```python
from build123d import *

# Parameters (mm, degrees)
SKETCH1_R           = 5
SKETCH1_R_2         = 1
BOSS_EXTRUDE1_DEPTH = 1
SKETCH3_R           = 6
BOSS_EXTRUDE2_DEPTH = 2
SKETCH4_R           = 5
CUT_EXTRUDE1_DEPTH  = 1
SKETCH5_R           = 4
CUT_EXTRUDE2_DEPTH  = 1
SKETCH6_R           = 3
BOSS_EXTRUDE3_DEPTH = 2
SKETCH7_R           = 1
CUT_EXTRUDE3_DEPTH  = 2


with BuildPart() as part:
    # Sketch1 → Boss-Extrude1 (new body)
    with BuildSketch(Plane(origin=(0, 0, 0), x_dir=(1, 0, 0), z_dir=(0, 1, 0))):
        with BuildLine():
            ThreePointArc((-4.117647059, 8.98545751), (-9.474873734, 9.474873734), (-8.98545751, 4.117647059))
            ThreePointArc((-8.98545751, 4.117647059), (-6.82182538, 0), (-8.98545751, -4.117647059))
            ThreePointArc((-8.98545751, -4.117647059), (-9.474873734, -9.474873734), (-4.117647059, -8.98545751))
            ThreePointArc((-4.117647059, -8.98545751), (0, -6.82182538), (4.117647059, -8.98545751))
            ThreePointArc((4.117647059, -8.98545751), (9.474873734, -9.474873734), (8.98545751, -4.117647059))
            ThreePointArc((8.98545751, -4.117647059), (6.82182538, 0), (8.98545751, 4.117647059))
            ThreePointArc((8.98545751, 4.117647059), (9.474873734, 9.474873734), (4.117647059, 8.98545751))
            ThreePointArc((4.117647059, 8.98545751), (0, 6.82182538), (-4.117647059, 8.98545751))
        make_face()
        with Locations(Location((0, 0, 0), (0, 0, 270))):
            Circle(SKETCH1_R, mode=Mode.SUBTRACT)
        with Locations(Location((-7, 7, 0), (0, 0, 270))):
            Circle(SKETCH1_R_2, mode=Mode.SUBTRACT)
        with Locations(Location((7, 7, 0), (0, 0, 270))):
            Circle(SKETCH1_R_2, mode=Mode.SUBTRACT)
        with Locations(Location((7, -7, 0), (0, 0, 270))):
            Circle(SKETCH1_R_2, mode=Mode.SUBTRACT)
        with Locations(Location((-7, -7, 0), (0, 0, 270))):
            Circle(SKETCH1_R_2, mode=Mode.SUBTRACT)
    extrude(amount=BOSS_EXTRUDE1_DEPTH)

    # Sketch3 → Boss-Extrude2 (add)
    with BuildSketch(Plane(origin=(0, 1, 0), x_dir=(1, 0, 0), z_dir=(0, 1, 0))):
        with Locations(Location((0, 0, 0), (0, 0, 270))):
            Circle(SKETCH3_R)
    extrude(amount=BOSS_EXTRUDE2_DEPTH)

    # Sketch4 → Cut-Extrude1 (cut)
    with BuildSketch(Plane.XZ.offset(-1)):
        with Locations(Location((0, 0, 0), (0, 0, 270))):
            Circle(SKETCH4_R)
    extrude(amount=-CUT_EXTRUDE1_DEPTH, mode=Mode.SUBTRACT)

    # Sketch5 → Cut-Extrude2 (cut)
    with BuildSketch(Plane.XZ.offset(-2)):
        with Locations(Location((0, 0, 0), (0, 0, 270))):
            Circle(SKETCH5_R)
    extrude(amount=-CUT_EXTRUDE2_DEPTH, mode=Mode.SUBTRACT)

    # Sketch6 → Boss-Extrude3 (add)
    with BuildSketch(Plane(origin=(0, 1, 0), x_dir=(1, 0, 0), z_dir=(0, 1, 0))):
        with Locations(Location((-7, 7, 0), (0, 0, 270))):
            Circle(SKETCH6_R)
        with Locations(Location((7, 7, 0), (0, 0, 270))):
            Circle(SKETCH6_R)
        with Locations(Location((7, -7, 0), (0, 0, 270))):
            Circle(SKETCH6_R)
        with Locations(Location((-7, -7, 0), (0, 0, 270))):
            Circle(SKETCH6_R)
    extrude(amount=BOSS_EXTRUDE3_DEPTH)

    # Sketch7 → Cut-Extrude3 (cut)
    with BuildSketch(Plane.XZ.offset(-1)):
        with Locations(Location((-7, 7, 0), (0, 0, 270))):
            Circle(SKETCH7_R)
        with Locations(Location((7, 7, 0), (0, 0, 270))):
            Circle(SKETCH7_R)
        with Locations(Location((7, -7, 0), (0, 0, 270))):
            Circle(SKETCH7_R)
        with Locations(Location((-7, -7, 0), (0, 0, 270))):
            Circle(SKETCH7_R)
    extrude(amount=-CUT_EXTRUDE3_DEPTH, mode=Mode.SUBTRACT)


solid = part.part
```
Design review of the part built by this model. Coordinates are the model's own, in mm. A direction names the side the tool comes from. Coordinates: 2 decimals unless noted, no trailing zeros. Loops run counter-clockwise (first coordinate to the right, second up) from the corner with the lowest first, then second, coordinate; pieces in that order, holes last. Notation, with made-up numbers: (82.25, -25.75) -> (108.25, -25.75) arc R12 cw to (108.25, -9.75) -> close; hole circle Ø5 at (86.5, 49). An arc over 180 degrees is marked (long way). Answer as a JSON object with one key per item and string values.
Q1. To check wall thickness, follow L1, parallel to X at y = 2.95, z = 7; L2, parallel to X at y = 2.35, z = 0; L3, parallel to Z at x = 6.75, y = 2.25. State the ranges of each line that lie inside material, in increasing order.
Answer block:
{"L1": "x = -10 to -8, -6 to -4, 4 to 6, 8 to 10", "L2": "x = -6 to -4, 4 to 6", "L3": "z = -9.99 to -7.97, -6.03 to -4.01, 4.01 to 6.03, 7.97 to 9.99"}
Q2. Take a section at A-A on y = 1.3. Give the number of separate pieces and of enclosed holes in the cut face, plus the area to 3 significant figures.
Answer block:
{"separate pieces": "5", "enclosed holes": "5", "area": "135 mm^2"}
Q3. Take a section at B-B on z = 0. Give the boundary of the cut face in (x, y).
Answer block:
{"outline": "(-6.82, 0) -> (-5, 0) -> (-5, 2) -> (-4, 2) -> (-4, 3) -> (-6, 3) -> (-6, 1) -> (-6.82, 1) -> close; (4, 2) -> (5, 2) -> (5, 0) -> (6.82, 0) -> (6.82, 1) -> (6, 1) -> (6, 3) -> (4, 3) -> close"}
Q4. The part is to be moulded in two halves that separate along Z. For faces 3 (the cylindrical face through (0.068, 0.493, -6.822)), 4 (the cylindrical face through (-3.905, 2.493, 0.867)), 5 (the flat face through (-6, 3, -8)), 6 (the cylindrical face through (-0.068, 0.493, 6.822)), say which applies: +Z half, -Z half, draft (parallel to the pull), parting line (faces both ways), or undercut.
Answer block:
{"face 3": "-Z half", "face 4": "undercut", "face 5": "draft", "face 6": "+Z half"}
Q5. Tool access review of faces 1 (the flat face through (-6, 3, 6)), 2 (the cylindrical face through (-6.1, 1.99, -4.14)): name each direction out of +Z, -Z, +X, -X, +Y, -Y from which nothing blocks a thin tool from reaching the whole face with its end or side.
Answer block:
{"face 1": "+Z, -Z, +X, -X, +Y", "face 2": "+Y"}
Q6. Clearance check with flat-ended pins moving along their axes: pin 1 Ø1.6 at (x, z) = (-7, -7) entering from +Y; pin 2 Ø11.5 at (x, z) = (0, 0) entering from +Y; pin 3 Ø5 at (x, z) = (0.5, -1.5) entering from -Y; pin 4 Ø1.5 at (y, z) = (2, -2) entering from -X. State where each tip first meets the part, or that it passes through.
Answer block:
{"pin 1": "passes through", "pin 2": "stops at y = 3", "pin 3": "stops at y = 2", "pin 4": "stops at x = -5.87"}
Q7. Take a section at C-C on x = 0. Give the boundary of the cut face in (y, z).
Answer block:
{"outline": "(0, -6.82) -> (1, -6.82) -> (1, -6) -> (3, -6) -> (3, -4) -> (2, -4) -> (2, -5) -> (0, -5) -> close; (0, 5) -> (2, 5) -> (2, 4) -> (3, 4) -> (3, 6) -> (1, 6) -> (1, 6.82) -> (0, 6.82) -> close"}
